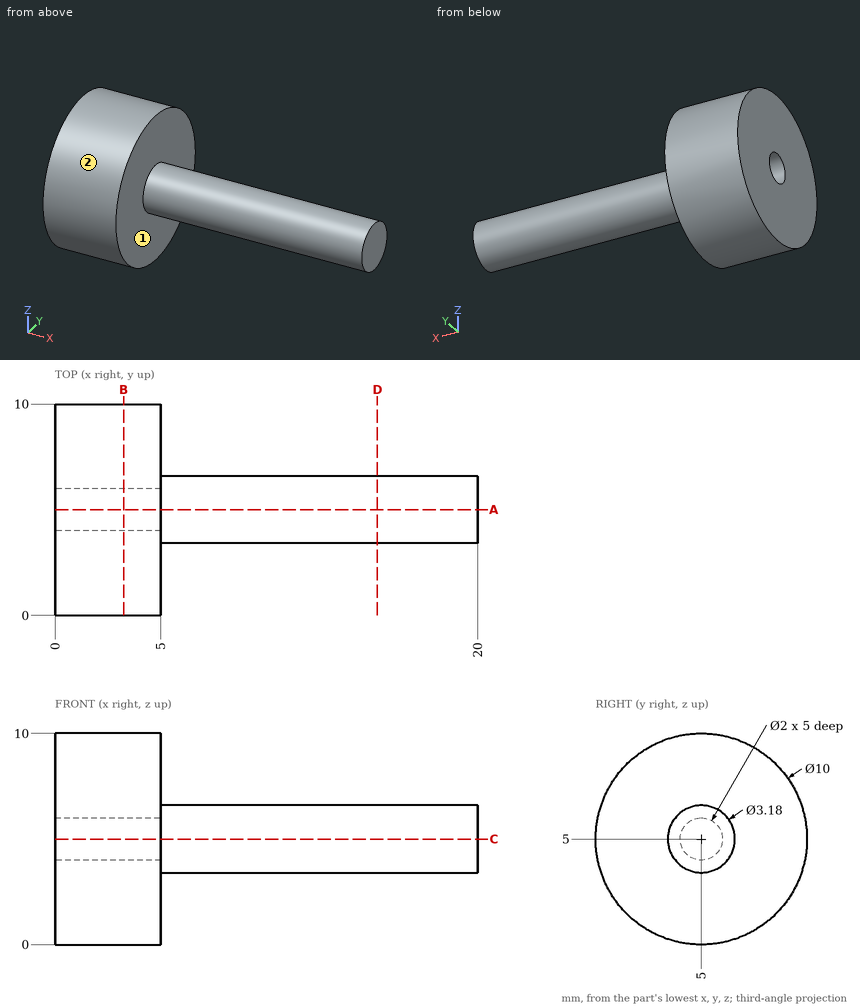
For this review, use the dimensioned drawing (mm, ordinates from the lowest corner) and the shaded views. A direction names the side the tool comes from. Give positions to 0.01 mm unless a question says otherwise; leave off trailing zeros. Write each loop counter-clockwise with the first axis right and the second up, starting at its lowest first coordinate (ties: lowest second). Pieces come first, ordered by that corner, then holes.
(1) Consider section A-A, the plane y = 5. Give the boundary of the cut face in (x, z), and give its area (3 significant figures).
(2) Consider section B-B, the plane x = 3.25. Give the boundary of the cut face in (y, z), and give its area (3 significant figures).
(3) For P1, Ø1.5, axis at y = 2, z = 4.5, coming from the +X side; P2, Ø3, axis at x = 12.5, z = 6, coming from the +Y side; P3, Ø2, axis at x = 4, z = 1, coming from the +Y side, all flat-tipped, find the tip position at first contact; note any pin that passes through.
(4) Tool access review of the marked faces 1 and 2: name each direction out of +Z, -Z, +X, -X, +Y, -Y from which nothing blocks a thin tool from reaching the whole face with its end or side.
(5) To check wall thickness, follow L1, parallel to Y at x = 1.5, z = 5; L2, parallel to X at y = 9.25, z = 4.5; L3, parallel to Z at x = 4, y = 7.5. State the ranges of each line that lie inside material, in increasing order.
(6) Consider section D-D, the plane x = 15.25. Give the boundary of the cut face in (y, z), and give its area (3 significant figures).
Returned:
1. outline: (0, 0) - (5, 0) - (5, 3.41) - (20, 3.41) - (20, 6.59) - (5, 6.59) - (5, 10) - (0, 10) - (0, 6) - (5, 6) - (5, 4) - (0, 4) - close
1. area: 87.7 mm2
2. outline: circle Ø10 at (5, 5); hole circle Ø2 at (5, 5)
2. area: 75.4 mm2
3. P1: stops at x = 5
3. P2: stops at y = 6.59
3. P3: stops at y = 9
4. face 1: +X
4. face 2: +X, -X
5. L1: y = 0 to 4, 6 to 10
5. L2: x = 0 to 5
5. L3: z = 0.67 to 9.33
6. outline: circle Ø3.18 at (5, 5)
6. area: 7.94 mm2
